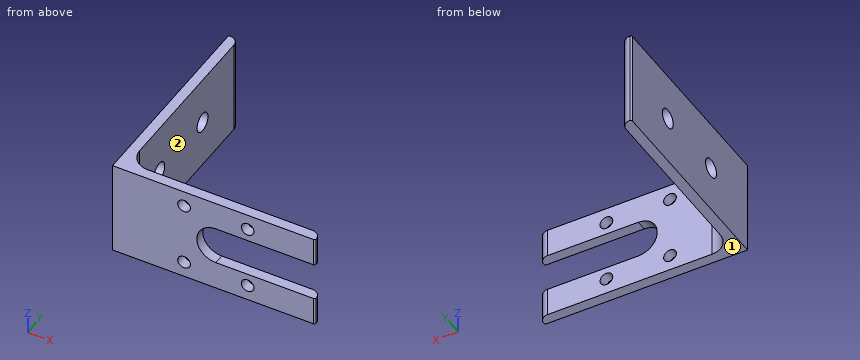
from build123d import *

# Parameters (mm, degrees)
BOSS_EXTRUDE1_DEPTH          = 30
F_4_0_4_DIAMETER_HOLE1_D     = 4
F_4_0_4_DIAMETER_HOLE1_DEPTH = 10
F_4_0_4_DIAMETER_HOLE1_TIP   = 1.201721238
CUT_EXTRUDE1_DEPTH           = 93.867176656
F_6_0_6_DIAMETER_HOLE1_D     = 6
F_6_0_6_DIAMETER_HOLE1_DEPTH = 10
F_6_0_6_DIAMETER_HOLE1_TIP   = 1.802581857


with BuildPart() as part:
    # Sketch2 → Boss-Extrude1 (new body)
    with BuildSketch(Plane.XY):
        with BuildLine():
            Line((0, 0), (63.26, 0))
            ThreePointArc((63.26, 0), (63.606482323, 0.143517677), (63.75, 0.49))
            Line((63.75, 0.49), (63.75, 0.5))
            ThreePointArc((63.75, 0.5), (62.944543648, 2.444543648), (61, 3.25))
            Line((61, 3.25), (9.25, 3.25))
            ThreePointArc((9.25, 3.25), (5.007359313, 5.007359313), (3.25, 9.25))
            Line((3.25, 9.25), (3.25, 61))
            ThreePointArc((3.25, 61), (2.444543648, 62.944543648), (0.5, 63.75))
            Line((0.5, 63.75), (0.49, 63.75))
            ThreePointArc((0.49, 63.75), (0.143517677, 63.606482323), (0, 63.26))
            Line((0, 63.26), (0, 0))
        make_face()
    extrude(amount=-BOSS_EXTRUDE1_DEPTH)

    # Ø4.0 (4) Diameter Hole1
    with Locations(Plane(origin=(0, 3.25, 0), x_dir=(1, 0, 0), z_dir=(0, 1, 0))):
        with Locations((22.5, 5), (22.5, 25), (42.5, 25), (42.5, 5)):
            Hole(F_4_0_4_DIAMETER_HOLE1_D / 2, depth=F_4_0_4_DIAMETER_HOLE1_DEPTH)
            with Locations((0, 0, -(F_4_0_4_DIAMETER_HOLE1_DEPTH + F_4_0_4_DIAMETER_HOLE1_TIP / 2))):  # 118° drill point
                Cone(0, F_4_0_4_DIAMETER_HOLE1_D / 2, F_4_0_4_DIAMETER_HOLE1_TIP, mode=Mode.SUBTRACT)

    # Sketch6 → Cut-Extrude1 (cut, through all)
    with BuildSketch(Plane(origin=(0, 3.25, 0), x_dir=(1, 0, 0), z_dir=(0, 1, 0))):
        with BuildLine():
            Line((32.5, 9), (66.86726804, 9))
            Line((66.86726804, 9), (66.86726804, 21))
            Line((66.86726804, 21), (32.5, 21))
            ThreePointArc((32.5, 21), (26.5, 15), (32.5, 9))
        make_face()
    extrude(amount=-CUT_EXTRUDE1_DEPTH, mode=Mode.SUBTRACT)

    # Ø6.0 (6) Diameter Hole1
    with Locations(Plane(origin=(3.25, 0, 0), x_dir=(0, 0, -1), z_dir=(1, 0, 0))):
        with Locations((15, 43.75), (15.399206183, 20)):
            Hole(F_6_0_6_DIAMETER_HOLE1_D / 2, depth=F_6_0_6_DIAMETER_HOLE1_DEPTH)
            with Locations((0, 0, -(F_6_0_6_DIAMETER_HOLE1_DEPTH + F_6_0_6_DIAMETER_HOLE1_TIP / 2))):  # 118° drill point
                Cone(0, F_6_0_6_DIAMETER_HOLE1_D / 2, F_6_0_6_DIAMETER_HOLE1_TIP, mode=Mode.SUBTRACT)


solid = part.part
Could you check a few things on this model? Use its own coordinates, in mm. Face numbers are marked on the shaded views. A direction names the side the tool comes from. Round coordinates to 2 decimals unless told otherwise and drop trailing zeros. Order: outer loops, then holes, each group sorted by start corner. A loop starts at its lowest first (then second) coordinate and runs counter-clockwise, first axis right, second up.
(1) I'm going to push flat-ended pins straight in: pin 1 (3 mm diameter, centred on y = 42, z = -9.5, fed in from +X); pin 2 (3 mm diameter, centred on x = 49.5, z = -22, fed in from +Y). Where does each tip first touch, or does it pass through?
Response values:
pin 1: stops at x = 3.25
pin 2: stops at y = 3.25
(2) Which directions (+Z, -Z, +X, -X, +Y, -Y) give clear straight access to the entire face, cutting with the end or side of a thin tool? Please do the marked faces 1 and 2.
Response values:
face 1: -Z, +X, -X, +Y, -Y
face 2: +Z, -Z, +X, +Y
(3) Imagine slicing it at A-A (z = -25). Count the separate pieces of the cut face and the enclosed holes in it, plus the area to 3 significant figures.
Response values:
separate pieces: 3
enclosed holes: 0
area: 382 mm2
(4) Imagine slicing it at B-B (x = 36). Write out the boundary of the cut face in (y, z).
Response values:
outline: (0, -30) - (3.25, -30) - (3.25, -21) - (0, -21) - close; (0, -9) - (3.25, -9) - (3.25, 0) - (0, 0) - close
(5) Please list where these lines run through material, in increasing order: line 1 along Z through (x, y) = (22.5, 2); line 2 along Z through (x, y) = (42.5, 0.75); line 3 along X through (y, z) = (0.8, -25).
Response values:
line 1: z = -30 to -27, -23 to -7, -3 to 0
line 2: z = -30 to -27, -23 to -21, -9 to -7, -3 to 0
line 3: x = 0 to 20.5, 24.5 to 40.5, 44.5 to 63.73
(6) Imagine slicing it at C-C (y = 20). Write out the boundary of the cut face in (x, z), plus the area to 3 significant figures.
Response values:
outline: (0, -30) - (3.25, -30) - (3.25, -18.4) - (0, -18.4) - close; (0, -12.4) - (3.25, -12.4) - (3.25, 0) - (0, 0) - close
area: 78.0 mm2
